```python
from build123d import *

# Parameters (mm, degrees)
SKETCH1_R           = 22.225
SKETCH1_R_2         = 0.9921875
SKETCH1_R_3         = 5.55625
BOSS_EXTRUDE1_DEPTH = 2.38125


with BuildPart() as part:
    # Sketch1 → Boss-Extrude1 (new body)
    with BuildSketch(Plane.XY):
        with Locations(Location((0, 0, 0), (0, 0, 180))):
            Circle(SKETCH1_R)
        with Locations(Location((-19.05, 0, 0), (0, 0, 180))):
            Circle(SKETCH1_R_2, mode=Mode.SUBTRACT)
        with Locations(Location((-13.470384182, 13.470384182, 0), (0, 0, 180))):
            Circle(SKETCH1_R_2, mode=Mode.SUBTRACT)
        with Locations(Location((0, 19.05, 0), (0, 0, 180))):
            Circle(SKETCH1_R_2, mode=Mode.SUBTRACT)
        with Locations(Location((13.470384182, 13.470384182, 0), (0, 0, 180))):
            Circle(SKETCH1_R_2, mode=Mode.SUBTRACT)
        with Locations(Location((19.05, 0, 0), (0, 0, 180))):
            Circle(SKETCH1_R_2, mode=Mode.SUBTRACT)
        with Locations(Location((13.470384182, -13.470384182, 0), (0, 0, 180))):
            Circle(SKETCH1_R_2, mode=Mode.SUBTRACT)
        with Locations(Location((0, -19.05, 0), (0, 0, 180))):
            Circle(SKETCH1_R_2, mode=Mode.SUBTRACT)
        with Locations(Location((-13.470384182, -13.470384182, 0), (0, 0, 180))):
            Circle(SKETCH1_R_2, mode=Mode.SUBTRACT)
        with Locations(Location((0, 0, 0), (0, 0, 180))):
            Circle(SKETCH1_R_3, mode=Mode.SUBTRACT)
    extrude(amount=BOSS_EXTRUDE1_DEPTH)


solid = part.part
```
The listing builds one solid part. Answer for the finished solid, in the listing's coordinates (mm). Give positions to 0.01 mm unless a question says otherwise; leave off trailing zeros. Write each loop counter-clockwise with the first axis right and the second up, starting at its lowest first coordinate (ties: lowest second). Pieces come first, ordered by that corner, then holes. Notation, with made-up numbers: (77, 38) - (82, 38) arc R25 cw to (82, 58) - close; hole circle Ø11 at (30, 52.25). An arc over 180 degrees is marked (long way). Use one line per item in the form item = value. Start each with the question number.
1) Find section A-A on y = 0. Determine the outline of the cut face in (x, z) (3 decimals).
2) Find section B-B on x = -19. Determine the outline of the cut face in (y, z).
3) Consider line 1 along Y through (x, z) = (0, 1.2) (3 decimals); line 2 along Y through (x, z) = (-13, 1.15); line 3 along X through (y, z) = (-19.05, 1.7). Determine where each line is inside the solid, lowest interval first. Write a range as from..to.
4) A flat-ended cylindrical pin translates along its axis: pin 1 Ø1 at (y, z) = (-6.5, 1.5) entering from -X. Find the tip coordinate at first contact, or state that the pin passes through.
5) Find section C-C on y = 19.05. Determine the outline of the cut face in (x, z), plus the area to 3 significant figures.
6) The mould has two halves that part along X. Classify faces 1 (the face through (13.01, 14.35, 1.17)), 2 (the face through (16.4, -15, 1.2)), 3 (the face through (-5, 5, 2.381)): pulls with the +X half, pulls with the -X half, needs draft (parallel to the pull), parting line crosses it, or undercut.
7) Find section D-D on z = 1.15. Count the separate pieces of the cut face and the enclosed holes in it, plus the area to 3 significant figures.
Geometry results:
q1.outline = (-22.225, 0) - (-20.042, 0) - (-20.042, 2.381) - (-22.225, 2.381) - close; (-18.058, 0) - (-5.556, 0) - (-5.556, 2.381) - (-18.058, 2.381) - close; (5.556, 0) - (18.058, 0) - (18.058, 2.381) - (5.556, 2.381) - close; (20.042, 0) - (22.225, 0) - (22.225, 2.381) - (20.042, 2.381) - close
q2.outline = (-11.53, 0) - (-0.99, 0) - (-0.99, 2.38) - (-11.53, 2.38) - close; (0.99, 0) - (11.53, 0) - (11.53, 2.38) - (0.99, 2.38) - close
q3.line_1 = -22.225..-20.042, -18.058..-5.556, 5.556..18.058, 20.042..22.225
q3.line_2 = -18.03..-14.34, -12.6..12.6, 14.34..18.03
q3.line_3 = -11.45..-0.99, 0.99..11.45
q4.pin_1 = -21.4
q5.outline = (-11.45, 0) - (-0.99, 0) - (-0.99, 2.38) - (-11.45, 2.38) - close; (0.99, 0) - (11.45, 0) - (11.45, 2.38) - (0.99, 2.38) - close
q5.area = 49.8 mm2
q6.face_1 = undercut
q6.face_2 = parting line crosses it
q6.face_3 = needs draft
q7.separate_pieces = 1
q7.enclosed_holes = 9
q7.area = 1,430 mm2
